Verification items for the finished model (mm, model axes). Face numbers are marked on the shaded views. A direction names the side the tool comes from. Give positions to 0.01 mm unless a question says otherwise; leave off trailing zeros. Order: outer loops, then holes, each group sorted by start corner. A loop starts at its lowest first (then second) coordinate and runs counter-clockwise, first axis right, second up. Notation, with made-up numbers: (76, 4) - (112, 4) arc R25 cw to (112, 25) - close; hole circle Ø2 at (-11.5, -15). An arc over 180 degrees is marked (long way). Answer as a JSON object with one key per item and string values. Group by question number.
(1) Access from +Z, -Z, +X, -X, +Y, -Y to the whole of each face (thin tool, end or side, straight path). Record for the marked faces 1, 2, 3, 4 and 5.
(2) Depth check by flat-ended pin: pin 1 Ø4 at (y, z) = (-26, 15.5) entering from +X; pin 2 Ø17 at (x, z) = (95, 35) entering from +Y; pin 3 Ø24 at (x, z) = (93.5, 30.5) entering from -Y. Enter the tip coordinate at first touch or a pass-through.
(3) Section check C-C (y = 6.5). Record the boundary of the cut face in (x, z), then the cut area to 3 significant figures.
(4) Mould release check, pull along Z, two halves, no side actions. Record for the marked faces 6, 7 and 8: +Z half, -Z half, draft (parallel to the pull), parting line (faces both ways), or undercut.
(5) Section check A-A (z = 35). Record the boundary of the cut face in (x, y), then the cut area to 3 significant figures.
(6) Section check D-D (y = -36.5). Record the boundary of the cut face in (x, z), then the cut area to 3 significant figures.
(7) Section check B-B (x = -84). Record the boundary of the cut face in (y, z), then the cut area to 3 significant figures.
(8) Thickness scan on line 1 (Z direction, x = -95, y = -7); line 2 (Y direction, x = 1.5, z = 45); line 3 (X direction, y = 11.5, z = 41.5). Record the ranges inside material, lowest first.
```python
from build123d import *

# Parameters (mm, degrees)
SKETCH_1_R               = 70
EXTRUDE_1_DEPTH          = 120
SKETCH_3_R               = 50
CUT_EXTRUDE_1_DEPTH      = 121
EXTRUDE_2_DEPTH          = 15
SKETCH_5_R               = 7.5
CUT_EXTRUDE_2_DEPTH      = 71
CUT_EXTRUDE_2_DEPTH_BACK = 71
SKETCH_6_R               = 50
CUT_EXTRUDE_3_DEPTH      = 121


with BuildPart() as part:
    # 스케치1 → 보스-돌출1 (new body)
    with BuildSketch(Plane.XY):
        Circle(SKETCH_1_R)
    extrude(amount=EXTRUDE_1_DEPTH)

    # 스케치3 → 컷-돌출1 (cut, through all)
    with BuildSketch(Plane.XY):
        Circle(SKETCH_3_R)
    extrude(amount=CUT_EXTRUDE_1_DEPTH, mode=Mode.SUBTRACT)

    # 스케치4 → 보스-돌출2 (add, symmetric)
    with BuildSketch(Plane(origin=(0, 0, 0), x_dir=(1, 0, 0), z_dir=(0, 1, 0))):
        with BuildLine():
            Line((-95, -20), (95, -20))
            ThreePointArc((95, -20), (110, -35), (95, -50))
            Line((95, -50), (-95, -50))
            ThreePointArc((-95, -50), (-110, -35), (-95, -20))
        make_face()
        with BuildLine():
            Line((-95, -100), (95, -100))
            ThreePointArc((95, -100), (110, -85), (95, -70))
            Line((95, -70), (-95, -70))
            ThreePointArc((-95, -70), (-110, -85), (-95, -100))
        make_face()
    extrude(amount=EXTRUDE_2_DEPTH, both=True)

    # 스케치5 → 컷-돌출2 (cut, two sides)
    with BuildSketch(Plane(origin=(0, 0, 0), x_dir=(1, 0, 0), z_dir=(0, 1, 0))) as cut_extrude_2_sk:
        with Locations((95, -35)):
            Circle(SKETCH_5_R)
        with Locations((95, -85)):
            Circle(SKETCH_5_R)
        with Locations((-95, -35)):
            Circle(SKETCH_5_R)
        with Locations((-95, -85)):
            Circle(SKETCH_5_R)
    extrude(amount=CUT_EXTRUDE_2_DEPTH, mode=Mode.SUBTRACT)
    extrude(cut_extrude_2_sk.sketch, amount=-CUT_EXTRUDE_2_DEPTH_BACK, mode=Mode.SUBTRACT)

    # 스케치6 → 컷-돌출3 (cut, through all)
    with BuildSketch(Plane.XY):
        Circle(SKETCH_6_R)
    extrude(amount=CUT_EXTRUDE_3_DEPTH, mode=Mode.SUBTRACT)


solid = part.part
```
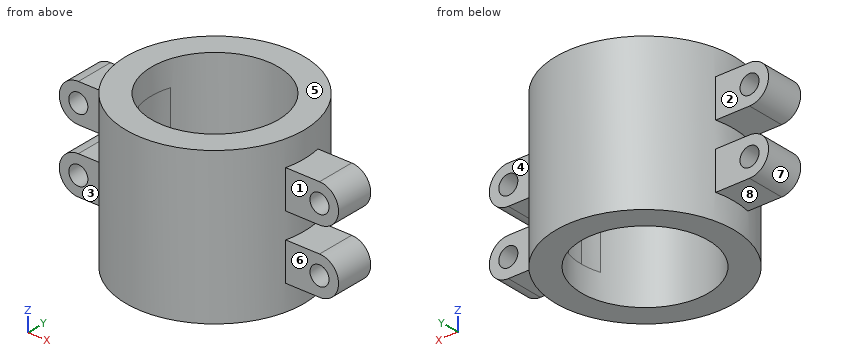
Solutions:
{
 "1": {"face 1": "+Z, -Z, +X, -Y", "face 2": "+Z, -Z, -X, +Y", "face 3": "+Z, -Z, -X, -Y", "face 4": "+Z, -Z, +X, +Y", "face 5": "+Z, +X, -X, +Y, -Y"},
 "2": {"pin 1": "stops at x = 65.76", "pin 2": "stops at y = 15", "pin 3": "stops at y = -15"},
 "3": {"outline": "(-95, 20) - (-69.7, 20) - (-69.7, 0) - (-49.58, 0) - (-49.58, 120) - (-69.7, 120) - (-69.7, 100) - (-95, 100) arc R15 ccw to (-95, 70) - (-69.7, 70) - (-69.7, 50) - (-95, 50) arc R15 ccw to start; (49.58, 0) - (69.7, 0) - (69.7, 20) - (95, 20) arc R15 ccw to (95, 50) - (69.7, 50) - (69.7, 70) - (95, 70) arc R15 ccw to (95, 100) - (69.7, 100) - (69.7, 120) - (49.58, 120) - close; hole circle Ø15 at (-95, 35); hole circle Ø15 at (-95, 85); hole circle Ø15 at (95, 35); hole circle Ø15 at (95, 85)", "area": "8,570 mm2"},
 "4": {"face 6": "draft", "face 7": "undercut", "face 8": "-Z half"},
 "5": {"outline": "(-110, -15) - (-102.5, -15) - (-102.5, 15) - (-110, 15) - close; (-87.5, -15) - (-68.37, -15) arc R70 ccw to (68.37, -15) - (87.5, -15) - (87.5, 15) - (68.37, 15) arc R70 ccw to (-68.37, 15) - (-87.5, 15) - close; (102.5, -15) - (110, -15) - (110, 15) - (102.5, 15) - close; hole circle Ø100 at (0, 0)", "area": "9,070 mm2"},
 "6": {"outline": "(-59.73, 0) - (-34.17, 0) - (-34.17, 120) - (-59.73, 120) - close; (34.17, 0) - (59.73, 0) - (59.73, 120) - (34.17, 120) - close", "area": "6,130 mm2"},
 "7": {"outline": "(-15, 20) - (15, 20) - (15, 50) - (-15, 50) - close; (-15, 70) - (15, 70) - (15, 100) - (-15, 100) - close", "area": "1,800 mm2"},
 "8": {"line 1": "z = 20 to 27.5, 42.5 to 50, 70 to 77.5, 92.5 to 100", "line 2": "y = -69.98 to -49.98, 49.98 to 69.98", "line 3": "x = -108.52 to -98.74, -91.26 to -48.66, 48.66 to 91.26, 98.74 to 108.52"}
}
